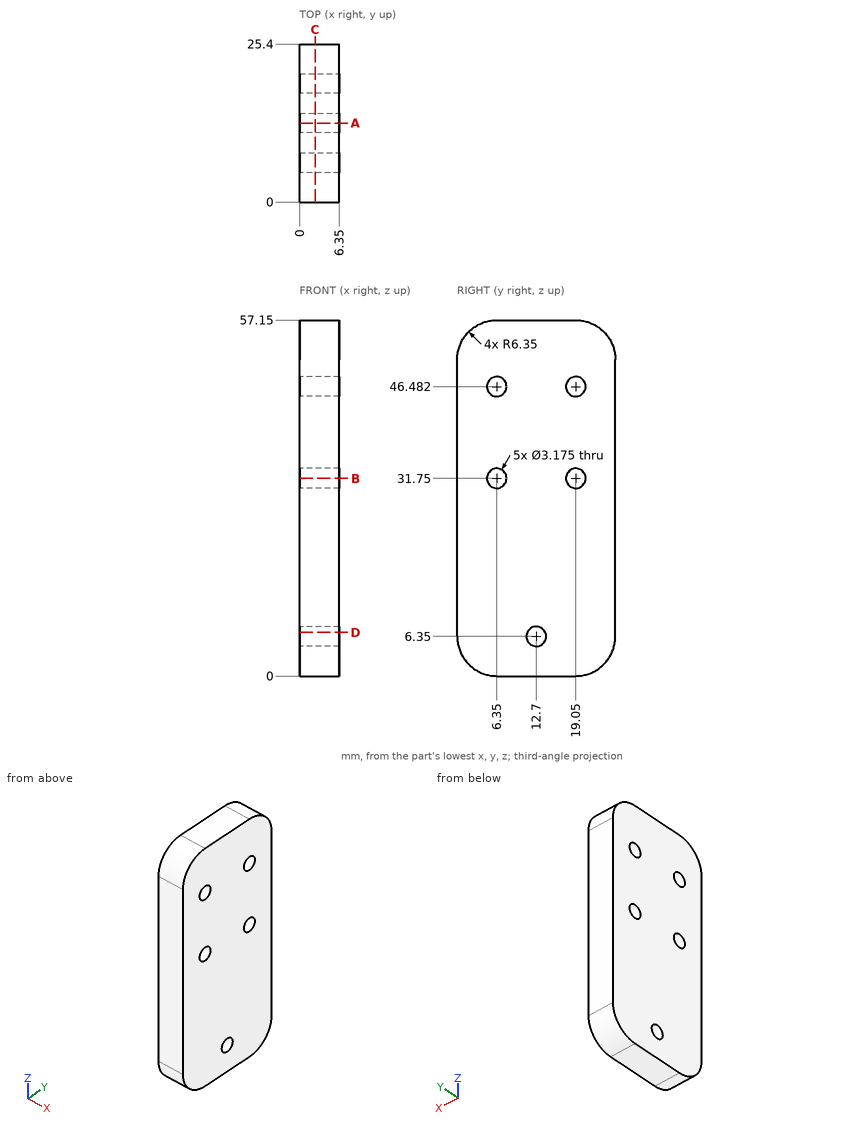
Job drawing, mm, ordinate dimensions from the low corner. One solid piece. Round coordinates to 2 decimals unless told otherwise and drop trailing zeros. Loops run counter-clockwise (first coordinate to the right, second up) from the corner with the lowest first, then second, coordinate; pieces in that order, holes last.
Item 1: Drop a flat-ended pin along its axis: P1, Ø1.9, axis at y = 6.35, z = 31.75, coming from the -X side. Give the stop position or say it passes through.
Item 2: Drill centre lines: line 1 (Z direction, x = 2.5, y = 6.35); line 2 (Z direction, x = 1.5, y = 12.7); line 3 (Z direction, x = 5, y = 6). Where is each one in solid material? Low to high.
Item 3: Cut at C-C, the plane x = 2.5. State how many separate pieces and enclosed holes the cut face has, then the cut area to 3 significant figures.
Item 4: Cut at B-B, the plane z = 31.75. Give the cut face in (x, y), then the cut area to 3 significant figures.
Item 5: Cut at D-D, the plane z = 7. Give the cut face in (x, y).
Item 6: Cut at A-A, the plane y = 12.7. Give the cut face in (x, z).
A:
1. P1: passes through
2. line 1: z = 0 to 30.16, 33.34 to 44.89, 48.07 to 57.15
2. line 2: z = 0 to 4.76, 7.94 to 57.15
2. line 3: z = 0.01 to 30.2, 33.3 to 44.93, 48.03 to 57.14
3. separate pieces: 1
3. enclosed holes: 5
3. area: 1,380 mm2
4. outline: (0, 0) - (6.35, 0) - (6.35, 4.76) - (0, 4.76) - close; (0, 7.94) - (6.35, 7.94) - (6.35, 17.46) - (0, 17.46) - close; (0, 20.64) - (6.35, 20.64) - (6.35, 25.4) - (0, 25.4) - close
4. area: 121 mm2
5. outline: (0, 0) - (6.35, 0) - (6.35, 11.25) - (0, 11.25) - close; (0, 14.15) - (6.35, 14.15) - (6.35, 25.4) - (0, 25.4) - close
6. outline: (0, 0) - (6.35, 0) - (6.35, 4.76) - (0, 4.76) - close; (0, 7.94) - (6.35, 7.94) - (6.35, 57.15) - (0, 57.15) - close
